The listing builds one solid part. Answer for the finished solid, in the listing's coordinates (mm). A direction names the side the tool comes from. Round coordinates to 2 decimals unless told otherwise and drop trailing zeros. Answer in a Markdown table with one row per item. Add a question column.
Autodesk Inventor part; units mm, degrees
ref_plane "YZ Plane" through (0, 0, 0) normal (1, 0, 0) x (0, 1, 0)
ref_plane "XZ Plane" through (0, 0, 0) normal (0, 1, 0) x (-1, 0, 0)
ref_plane "XY Plane" through (0, 0, 0) normal (0, 0, 1) x (1, 0, 0)
ref_plane "작업 평면1" through (-380, -430.4083, 1686.95) normal (1, 0, 0) x (0, 1, 0)
sketch "스케치1" plane through (-380, -430.4083, 1686.95) normal (1, 0, 0) x (0, 1, 0)
  circle A0 centre (0, 0) radius 290
  point P0 (430.4083, -1686.95)
  dimension "d0" = 580
extrude "돌출1" add sketch "스케치1" along normal blind 100
sketch "스케치3" plane through (-280, -430.4083, 1686.95) normal (1, 0, 0) x (0, 0, -1)
  circle A0 centre (0, 0) radius 225
  circle A1 centre (0, 0) radius 20
  circle A2 centre (0, 0) radius 50
  arc A3 (225, 0) -> (50, 0) centre (137.5, -121.8349) ccw
  arc A4 (0, -225) -> (0, -50) centre (-121.8349, -137.5) ccw
  line L0 (0, 0) -> (159.099, -159.099)
  line L1 (0, 0) -> (225, 0) construction
  line L2 (159.099, -159.099) -> (-159.099, 159.099)
  line L3 (0, 0) -> (159.099, 159.099)
  line L4 (0, 0) -> (225, 0) construction
  line L5 (159.099, 159.099) -> (-159.099, -159.099)
  arc A5 (-159.099, -159.099) -> (-35.3553, -35.3553) centre (-183.3775, -11.0769) ccw
  arc A6 (159.099, 159.099) -> (35.3553, 35.3553) centre (183.3775, 11.0769) ccw
  arc A7 (159.099, -159.099) -> (35.3553, -35.3553) centre (11.0769, -183.3775) ccw
  arc A8 (-225, 0) -> (-50, 0) centre (-137.5, 121.8349) ccw
  arc A9 (-159.099, 159.099) -> (-35.3553, 35.3553) centre (-11.0769, 183.3775) ccw
  arc A10 (0, 225) -> (0, 50) centre (121.8349, 137.5) ccw
  point P0 (1686.95, 430.4083)
  dimension "d6" = 450
  dimension "d7" = 100
  dimension "d10" = 150
  dimension "d11" = 150
  dimension "d12" = 45
  dimension "d13" = 45
  dimension "d14" = 150
  dimension "d16" = 150
  dimension "d17" = 150
  dimension "d18" = 150
  dimension "d19" = 150
  dimension "d20" = 150
extrude "돌출3" cut sketch "스케치3" against normal blind 100 contours A0 A7 A2 A3 | A6 A2 A10 A0 | A0 A5 A2 A4 | A9 A2 A8 A0
fillet "모깎기1" radius 121.75 4 edges at (-330, -380.4083, 1686.95) (-330, -430.4083, 1736.95) (-330, -480.4083, 1686.95) (-330, -430.4083, 1636.95)
fillet "모깎기2" radius 36.25 4 edges at (-330, -205.4083, 1686.95) (-330, -430.4083, 1911.95) (-330, -430.4083, 1461.95) (-330, -655.4083, 1686.95)
sketch "스케치4" plane through (-280, -430.4083, 1686.95) normal (1, 0, 0) x (0, 0, -1)
  circle A0 centre (0, 0) radius 20
  point P0 (1686.95, 430.4083)
  dimension "d25" = 40
extrude "돌출4" add sketch "스케치4" along normal blind 5
properties part number "바퀴"
1. Each of these flat-tipped pins is pushed along its axis until it touches: pin 1 (2 mm diameter, centred on x = -332.5, y = -232, fed in from +Z); pin 2 (3 mm diameter, centred on x = -293, y = -589, fed in from -Z); pin 3 (10 mm diameter, centred on x = -323, z = 1868, fed in from -Y). Where does it stop, or does it pass through?
2. The part is cut by section A-A (x = -361.5). Give the number of separate pieces and of enclosed holes in the cut face, then the cut area to 3 significant figures.
3. The mould has two halves that part along Y. Classify faces 1 (the cylindrical face through (-329.3, -508.649, 1568.886)), 2 (the flat face through (-380, -434, 1691)), 3 (the cylindrical face through (-330.7, -296.59, 1944.23)): released by +Y, released by -Y, zero draft, split by the parting line, or undercut.
4. For faces 4 (the cylindrical face through (-329.3, -617.76, 1667.31)), 5 (the cylindrical face through (-277.535, -436.416, 1667.874)), 6 (the flat face through (-275, -430, 1687)), determine the directions among +Z, -Z, +X, -X, +Y, -Y from which every point of the face is accessible in a straight line to the end or side of a thin tool.
5. Straight lines are drawn through the part: line 1 along Z through (x, y) = (-287, -573.5); line 2 along Y through (x, z) = (-307, 1563); line 3 along Z through (x, y) = (-301.5, -492.5). For each, find the intervals that lie inside material, in ascending order.
Report:
| question | item | result |
|---|---|---|
| 1 | pin 1 | stops at z = 1899.39 |
| 1 | pin 2 | stops at z = 1443.18 |
| 1 | pin 3 | stops at y = -660.86 |
| 2 | separate pieces | 1 |
| 2 | enclosed holes | 4 |
| 2 | area | 191,000 mm^2 |
| 3 | face 1 | undercut |
| 3 | face 2 | zero draft |
| 3 | face 3 | split by the parting line |
| 4 | face 4 | +X, -X |
| 4 | face 5 | +X |
| 4 | face 6 | +Z, -Z, +X, +Y, -Y |
| 5 | line 1 | z = 1434.71 to 1513.31, 1531.38 to 1659.45, 1799.11 to 1939.19 |
| 5 | line 2 | y = -692.58 to -514.99, -404.5 to -281.61, -242.63 to -168.23 |
| 5 | line 3 | z = 1403.68 to 1470.69, 1587.61 to 1690.74, 1729.27 to 1970.22 |
